from build123d import *

# Parameters (mm, degrees)
SKETCH1_W           = 30
SKETCH1_H           = 11.5
SKETCH1_R           = 2.5
BOSS_EXTRUDE1_DEPTH = 3.5
SKETCH2_W           = 10
SKETCH2_H           = 11.5
BOSS_EXTRUDE2_DEPTH = 4.5
SKETCH3_W           = 2
SKETCH3_H           = 3.5
CUT_EXTRUDE1_DEPTH  = 23.29489852
SKETCH4_W           = 2
SKETCH4_H           = 3.5
CUT_EXTRUDE2_DEPTH  = 10
FILLET2_R           = 0.6


with BuildPart() as part:
    # Sketch1 → Boss-Extrude1 (new body)
    with BuildSketch(Plane.XY):
        Rectangle(SKETCH1_W, SKETCH1_H)
        with Locations((-10, -0.25)):
            Circle(SKETCH1_R, mode=Mode.SUBTRACT)
        with Locations((10, -0.25)):
            Circle(SKETCH1_R, mode=Mode.SUBTRACT)
    extrude(amount=BOSS_EXTRUDE1_DEPTH)

    # Sketch2 → Boss-Extrude2 (add)
    with BuildSketch(Plane.XY.offset(3.5)):
        Rectangle(SKETCH2_W, SKETCH2_H)
    extrude(amount=BOSS_EXTRUDE2_DEPTH)

    # Sketch3 → Cut-Extrude1 (cut, through all)
    with BuildSketch(Plane.ZY.offset(5)):
        with Locations((7, 4)):
            Rectangle(SKETCH3_W, SKETCH3_H)
    extrude(amount=-CUT_EXTRUDE1_DEPTH, mode=Mode.SUBTRACT)

    # Sketch4 → Cut-Extrude2 (cut)
    with BuildSketch(Plane.ZY.offset(5)):
        with Locations((7, -1)):
            Rectangle(SKETCH4_W, SKETCH4_H)
        with Locations((7, -6)):
            Rectangle(SKETCH4_W, SKETCH4_H)
    extrude(amount=-CUT_EXTRUDE2_DEPTH, mode=Mode.SUBTRACT)

    # Fillet2
    fillet2_edges = [part.edges().sort_by_distance(p)[0] for p in [
        (0, 2.25, 6),
        (0, -2.75, 6),
        (0, 0.75, 6),
        (0, -4.25, 6),
    ]]
    fillet(fillet2_edges, radius=FILLET2_R)


solid = part.part
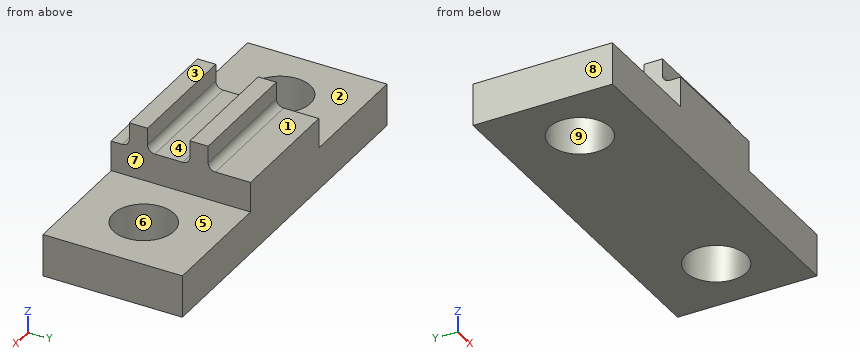
Verification items for the finished model (mm, model axes). Face numbers are marked on the shaded views. A direction names the side the tool comes from. Give positions to 0.01 mm unless a question says otherwise; leave off trailing zeros. Order: outer loops, then holes, each group sorted by start corner. A loop starts at its lowest first (then second) coordinate and runs counter-clockwise, first axis right, second up. Notation, with made-up numbers: M -0.5,7.25 L 55.5,7.25 A32 cw 55.5,33.25 Z; hole C 44.5,-20 d6. An arc over 180 degrees is marked long. Answer as a JSON object with one key per item and string values. Group by question number.
1) Access from +Z, -Z, +X, -X, +Y, -Y to the whole of each face (thin tool, end or side, straight path). Record for the marked faces 1, 2, 3, 4 and 5.
2) Cross-section at A-A (x = -10). Enter the section's corners in (y, z).
3) Cross-section at C-C (z = 7.25). Enter the section's corners in (x, y), then the cut area to 3 significant figures.
4) Depth check by flat-ended pin: pin 1 Ø4.5 at (x, y) = (-10, -0.25) entering from +Z; pin 2 Ø0.7 at (x, z) = (1, 7.5) entering from -Y; pin 3 Ø0.9 at (x, y) = (-2.5, 4.5) entering from +Z; pin 4 Ø0.7 at (x, z) = (1, 7.5) entering from +Y. Enter the tip coordinate at first touch or a pass-through.
5) Cross-section at B-B (y = -0.25). Enter the section's corners in (x, z), then the cut area to 3 significant figures.
6) Mould release check, pull along X, two halves, no side actions. Record for the marked faces 6, 7, 8 and 9: released by +X, released by -X, zero draft, split by the parting line, or undercut.
7) Scan lines: line 1 along Y through (x, z) = (-10, 1.55); line 2 along X through (y, z) = (4.5, 5); line 3 along Y through (x, z) = (1, 7.25). Record each from-to range of solid material in increasing order. Write a range as [from, to].
8) Cross-section at D-D (z = 3). Enter the section's corners in (x, y), then the cut area to 3 significant figures.
Result sheet:
{
 "1": {"face 1": "+Z, +X, -X, +Y", "face 2": "+Z, -X, +Y, -Y", "face 3": "+Z, +X, -X, +Y, -Y", "face 4": "+Z, +X, -X", "face 5": "+Z, +X, +Y, -Y"},
 "2": {"outline": "M -5.75,0 L -2.75,0 L -2.75,3.5 L -5.75,3.5 Z; M 2.25,0 L 5.75,0 L 5.75,3.5 L 2.25,3.5 Z"},
 "3": {"outline": "M -5,-4.25 L 5,-4.25 L 5,-2.75 L -5,-2.75 Z; M -5,0.75 L 5,0.75 L 5,2.25 L -5,2.25 Z", "area": "30.0 mm2"},
 "4": {"pin 1": "passes through", "pin 2": "stops at y = -4.25", "pin 3": "stops at z = 6", "pin 4": "stops at y = 2.25"},
 "5": {"outline": "M -15,0 L -12.5,0 L -12.5,3.5 L -15,3.5 Z; M -7.5,0 L 7.5,0 L 7.5,3.5 L 5,3.5 L 5,6 L -5,6 L -5,3.5 L -7.5,3.5 Z; M 12.5,0 L 15,0 L 15,3.5 L 12.5,3.5 Z", "area": "95.0 mm2"},
 "6": {"face 6": "undercut", "face 7": "released by +X", "face 8": "released by -X", "face 9": "undercut"},
 "7": {"line 1": "y = [-5.75, -2.75], [2.25, 5.75]", "line 2": "x = [-5, 5]", "line 3": "y = [-4.25, -2.75], [0.75, 2.25]"},
 "8": {"outline": "M -15,-5.75 L 15,-5.75 L 15,5.75 L -15,5.75 Z; hole C -10,-0.25 d5; hole C 10,-0.25 d5", "area": "306 mm2"}
}
